Could you check a few things on this model? Use its own coordinates, in mm. A direction names the side the tool comes from. Round coordinates to 2 decimals unless told otherwise and drop trailing zeros. Loops run counter-clockwise (first coordinate to the right, second up) from the corner with the lowest first, then second, coordinate; pieces in that order, holes last. Notation, with made-up numbers: M 79,83.25 L 118,83.25 A11 cw 118,89.25 Z; hole C -33.5,10.25 d7. An arc over 180 degrees is marked long. Return JSON: item names as keys, results as strings. Group by question number.
```python
from build123d import *

# Parameters (mm, degrees)
F0_W           = 20
F0_H           = 80
F1_DEPTH       = 3
F5_D           = 5.5
F5_DEPTH       = 15
F5_CSINK_D     = 8
F5_CSINK_ANGLE = 90
F5_TIP         = 1.6523667023
F7_R           = 0.5
F10_DEPTH      = 28


# Not quite as in the source:
# - two fillets or chamfers of one size are made in one step


with BuildPart() as f1:
    # F0 (on Top) → F1 (new body)
    with BuildSketch(Plane.XY):
        with Locations((0, 24)):
            Rectangle(F0_W, F0_H)
    extrude(amount=F1_DEPTH)

    # F5
    with Locations(Plane.XY.offset(3)):
        with Locations((0, 0), (0, 48)):
            CounterSinkHole(F5_D / 2, F5_CSINK_D / 2, depth=F5_DEPTH, counter_sink_angle=F5_CSINK_ANGLE)
            with Locations((0, 0, -(F5_DEPTH + F5_TIP / 2))):  # 118° drill point
                Cone(0, F5_D / 2, F5_TIP, mode=Mode.SUBTRACT)

    # F7
    f7_edges = [f1.edges().sort_by_distance(p)[0] for p in [
        (0, 64, 3),
        (-10, 24, 3),
        (10, 24, 3),
        (-10, -16, 1.5),
        (-10, 64, 1.5),
        (10, 64, 1.5),
        (10, -16, 1.5),
        (0, -16, 3),
    ]]
    fillet(f7_edges, radius=F7_R)

    # F9 (on offset) → F10 (join)
    with BuildSketch(Plane.XZ.offset(-10)):
        with BuildLine():
            ThreePointArc((13, 3), (7.5, 3.860863499), (2, 3))
            Line((2, 3), (10, 3))
            Line((10, 3), (13, 3))
        make_face()
        with BuildLine():
            Line((0, 3), (2, 3))
            ThreePointArc((2, 3), (7.5, 3.860863499), (13, 3))
            Line((13, 3), (15, 3))
            ThreePointArc((15, 3), (7.5, 4.4595037823), (0, 3))
        make_face()
    extrude(amount=-F10_DEPTH)


solid = f1.part
```
1. We'd pull the mould along Y, two halves only. Please class faces 1 (the face through (0, 64, 1)), 2 (the face through (0.358, 50.727, 0.863)), 3 (the face through (10, 23, 1)): +Y half, -Y half, draft (parallel to the pull), parting line (faces both ways), or undercut.
2. If we section it at D-D, the plane z = 3.7: Please give me the cut outline in (x, y), then the cut area to 3 significant figures.
3. If we section it at C-C, the plane x = 10.75: Please give me the cut outline in (y, z).
4. I'm going to push flat-ended pins straight in: pin 1 Ø1.5 at (y, z) = (19, 1.5) entering from +X; pin 2 Ø0.7 at (x, z) = (7.5, 4) entering from +Y; pin 3 Ø3.5 at (x, y) = (0, 48) entering from +Z; pin 4 Ø12 at (x, y) = (-2, 37) entering from +Z. Where does each tip first touch, or does it pass through?
5. If we section it at A-A, the plane y = 0: Please give me the cut outline in (x, z), then the cut area to 3 significant figures.
6. I need wall thicknesses on probe 1 along Y at (x, z) = (0, 1.05); probe 2 along X at (y, z) = (48, 0.55); probe 3 along Y at (x, z) = (-0.5, 2). Which ranges of each line are inside material? Lowest first, please.
7. If we section it at B-B, the plane y = 19: Please give me the cut outline in (x, z), then the cut area to 3 significant figures.
8. On a 3-axis mill with a long thin cutter (end or side, diameter ignored), from which of +Z, -Z, +X, -X, +Y, -Y can I reach the whole of each face in a straight line? I mean faces 4 (the face through (7, 10, 4)), 5 (the face through (7, 38, 4)), 6 (the face through (-2, 25, 3)). Say none if no direction works.
Geometry results:
{
 "1": {"face 1": "+Y half", "face 2": "undercut", "face 3": "draft"},
 "2": {"outline": "M 2.04,10 L 12.96,10 L 12.96,38 L 2.04,38 Z", "area": "306 mm^2"},
 "3": {"outline": "M 10,3 L 38,3 L 38,4.19 L 10,4.19 Z"},
 "4": {"pin 1": "x = 10", "pin 2": "y = 38", "pin 3": "through", "pin 4": "z = 4.15"},
 "5": {"outline": "M -10,0 L -2.75,0 L -2.75,1.75 L -4,3 L -9.5,3 A0.5 ccw -10,2.5 Z; M 2.75,0 L 10,0 L 10,2.5 A0.5 ccw 9.5,3 L 4,3 L 2.75,1.75 Z", "area": "41.8 mm^2"},
 "6": {"probe 1": "-16 to -2.75, 2.75 to 45.25, 50.75 to 64", "probe 2": "-10 to -2.75, 2.75 to 10", "probe 3": "-16 to -2.96, 2.96 to 45.04, 50.96 to 64"},
 "7": {"outline": "M -10,0 L 10,0 L 10,2.5 A0.5 ccw 9.5,3 L 15,3 A20 ccw 0,3 L -9.5,3 A0.5 ccw -10,2.5 Z", "area": "74.6 mm^2"},
 "8": {"face 4": "+Z, +X, -X, -Y", "face 5": "+Z, +X, -X, +Y", "face 6": "+Z, -X"}
}
